from build123d import *

# Parameters (mm, degrees)
BOSS_EXTRU_1_DEPTH = 2.5
ESQUISSE3_R        = 0.375
BOSS_EXTRU_2_DEPTH = 6
CHANFREIN1_SIZE    = 0.25
BOSS_EXTRU_3_DEPTH = 0.2
CONG_1_R           = 0.15
CONG_2_R           = 0.15


with BuildPart() as part:
    # Esquisse1 → Boss.-Extru.1 (new body)
    with BuildSketch(Plane(origin=(0, 0, 0), x_dir=(1, 0, 0), z_dir=(0, 1, 0))):
        with BuildLine():
            Line((-1.25, 1.05), (-1.446931313, 1.05))
            Line((-1.446931313, 1.05), (-1.446931313, -1.05))
            Line((-1.446931313, -1.05), (-1.25, -1.05))
            ThreePointArc((-1.25, -1.05), (-1.191421356, -1.191421356), (-1.05, -1.25))
            Line((-1.05, -1.25), (1.05, -1.25))
            ThreePointArc((1.05, -1.25), (1.191421356, -1.191421356), (1.25, -1.05))
            Line((1.25, -1.05), (1.449962609, -1.05))
            Line((1.449962609, -1.05), (1.449962609, 1.05))
            Line((1.449962609, 1.05), (1.25, 1.05))
            ThreePointArc((1.25, 1.05), (1.191421356, 1.191421356), (1.05, 1.25))
            Line((1.05, 1.25), (-1.05, 1.25))
            ThreePointArc((-1.05, 1.25), (-1.191421356, 1.191421356), (-1.25, 1.05))
        make_face()
    extrude(amount=BOSS_EXTRU_1_DEPTH)

    # Esquisse3 → Boss.-Extru.2 (add)
    with BuildSketch(Plane(origin=(0, 2.5, 0), x_dir=(1, 0, 0), z_dir=(0, 1, 0))):
        with Locations(Location((0, 0, 0), (0, 0, 90))):
            Circle(ESQUISSE3_R)
    extrude(amount=BOSS_EXTRU_2_DEPTH)

    # Chanfrein1
    chanfrein1_edges = [part.edges().sort_by_distance(p)[0] for p in [
        (0, 8.5, 0.375),
    ]]
    chamfer(chanfrein1_edges, length=CHANFREIN1_SIZE)

    # Esquisse4 → Boss.-Extru.3 (add)
    with BuildSketch(Plane.XZ):
        Polygon((0, 0), (0.304241832, 0), (0.304241832, -2.250938438), (0, -2.250938438), (-0.299312937, -2.250938438), (-0.299312937, 0), align=None)
    extrude(amount=BOSS_EXTRU_3_DEPTH)

    # Congé1
    cong_1_edges = [part.edges().sort_by_distance(p)[0] for p in [
        (0.002464447, 0, -2.250938438),
    ]]
    fillet(cong_1_edges, radius=CONG_1_R)

    # Congé2
    cong_2_edges = [part.edges().sort_by_distance(p)[0] for p in [
        (-0.299312937, 0, -1.675469219),
        (-0.299312937, -0.175, -2.250938438),
        (0.304241832, -0.175, -2.250938438),
        (0.304241832, 0, -1.675469219),
        (0.304241832, -0.043933983, -2.207004455),
        (-0.299312937, -0.043933983, -2.207004455),
    ]]
    fillet(cong_2_edges, radius=CONG_2_R)


solid = part.part
The listing builds one solid part. Answer for the finished solid, in the listing's coordinates (mm). A direction names the side the tool comes from. Give positions to 0.01 mm unless a question says otherwise; leave off trailing zeros. Write each loop counter-clockwise with the first axis right and the second up, starting at its lowest first coordinate (ties: lowest second). Pieces come first, ordered by that corner, then holes.
Item 1: Flat-ended cylindrical pins translate along their axes: P1, Ø1.7, axis at x = 0.5, y = 1.5, coming from the -Z side; P2, Ø0.8, axis at x = -0.5, z = -0.5, coming from the +Y side; P3, Ø2, axis at y = 6, z = 0.5, coming from the -X side (3 decimals); P4, Ø1.5, axis at x = -0.5, z = 0, coming from the +Y side. Find the tip coordinate at first contact, or state that the pin passes through.
Item 2: Which of the six approach directions +Z, -Z, +X, -X, +Y, -Y give full straight-line access (tool end or side, diameter ignored) to faces 1 (the flat face through (0, 1, 1.25)), 2 (the flat face through (0, 2.5, -1))?
Item 3: Section A-A, the plane z = -0.85 is taken. Write down the section's boundary in (x, y), plus the area to 3 significant figures.
Item 4: Section B-B, the plane x = 0 is taken. Write down the section's boundary in (y, z) (3 decimals).
Item 5: Section D-D, the plane z = -1.9 is taken. Write down the section's boundary in (x, y).
Item 6: Find the intervals of material crossed by line 1 along Z through (x, y) = (0.45, 1.25); line 2 along X through (y, z) = (5.5, 0) (3 decimals); line 3 along Y through (x, z) = (-0.25, 0.95), in increasing order.
Item 7: Section C-C, the plane y = 0.5 is taken. Write down the section's boundary in (x, z).
Completed:
1. P1: stops at z = -1.25
1. P2: stops at y = 8.32
1. P3: stops at x = -0.375
1. P4: stops at y = 8.5
2. face 1: +Z, +X, -X, +Y, -Y
2. face 2: +Y
3. outline: (-1.45, 0) - (-0.3, 0) - (-0.3, -0.2) - (0.3, -0.2) - (0.3, 0) - (1.45, 0) - (1.45, 2.5) - (-1.45, 2.5) - close
3. area: 7.36 mm2
4. outline: (-0.2, -2.251) - (-0.15, -2.251) arc R0.15 ccw to (0, -2.101) - (0, -1.25) - (2.5, -1.25) - (2.5, -0.375) - (8.25, -0.375) - (8.5, -0.125) - (8.5, 0.125) - (8.25, 0.375) - (2.5, 0.375) - (2.5, 1.25) - (0, 1.25) - (0, 0) - (-0.2, 0) - close
5. outline: (-0.3, -0.2) - (0.3, -0.2) - (0.3, -0.15) arc R0.15 ccw to (0.15, 0) - (-0.15, 0) arc R0.15 ccw to (-0.3, -0.15) - close
6. line 1: z = -1.25 to 1.25
6. line 2: x = -0.375 to 0.375
6. line 3: y = 0 to 2.5
7. outline: (-1.45, -1.05) - (-1.25, -1.05) arc R0.2 ccw to (-1.05, -1.25) - (1.05, -1.25) arc R0.2 ccw to (1.25, -1.05) - (1.45, -1.05) - (1.45, 1.05) - (1.25, 1.05) arc R0.2 ccw to (1.05, 1.25) - (-1.05, 1.25) arc R0.2 ccw to (-1.25, 1.05) - (-1.45, 1.05) - close
